Geometry check sheet. Reference: drawing and pictorial views, mm from the part's lowest x, y, z. A direction names the side the tool comes from. Coordinates: 2 decimals unless noted, no trailing zeros. Loops run counter-clockwise (first coordinate to the right, second up) from the corner with the lowest first, then second, coordinate; pieces in that order, holes last. Notation, with made-up numbers: (47.5, 59) -> (55.5, 59) arc R8 cw to (55.5, 70) -> close; hole circle Ø10 at (30, 75). An arc over 180 degrees is marked (long way). Answer as a JSON object with one key per item and string values. Group by question number.
Q1. Cross-section at A-A on y = 7. Give the number of separate pieces and of enclosed holes in the cut face, and give its area (3 significant figures).
Q2. Gauge pin test, flat ends, axial feed: pin 1 Ø2 at (x, z) = (3, 6) entering from -Y; pin 2 Ø6.5 at (x, y) = (5.5, 13.5) entering from -Z; pin 3 Ø2.5 at (y, z) = (17.5, 5.5) entering from +X; pin 4 Ø2 at (y, z) = (10, 2) entering from -X. Record the tip position at first contact, or that the pin passes through.
Q3. Set-up check for the marked faces 1 and 2: record each of +Z, -Z, +X, -X, +Y, -Y from which the full face is reachable in a straight line by a thin tool's end or side.
Q4. Cross-section at C-C on x = 3. Record the boundary of the cut face in (y, z).
Q5. Cross-section at B-B on z = 1. Record the boundary of the cut face in (x, y), and give its area (3 significant figures).
Q6. Cross-section at D-D on x = 9.5. Record the boundary of the cut face in (y, z), and give its area (3 significant figures).
Q7. Scan lines: L1, parallel to Y at x = 16.25, z = 4.75; L2, parallel to Z at x = 13, y = 19.65; L3, parallel to X at y = 7, z = 7. Record each from-to range of solid material in increasing order.
Q8. Release check for a two-part mould opening along Z. For the marked faces 3, 4 and 5 record: released by +Z, released by -Z, zero draft, split by the parting line, or undercut.
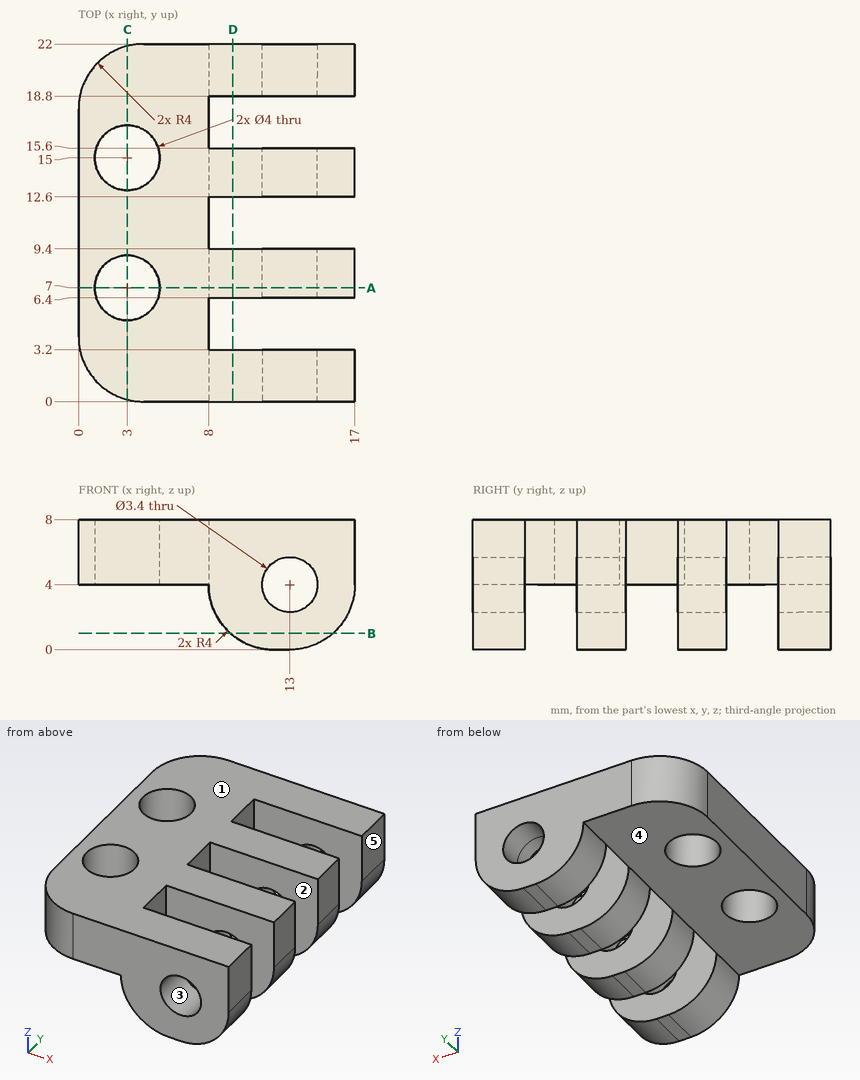
Computed values:
{
 "1": {"separate pieces": "2", "enclosed holes": "1", "area": "72.1 mm²"},
 "2": {"pin 1": "stops at y = 0", "pin 2": "stops at z = 1.67", "pin 3": "stops at x = 8", "pin 4": "stops at x = 8.18"},
 "3": {"face 1": "+Z, +X, -X, +Y, -Y", "face 2": "+Z, -Z, +X"},
 "4": {"outline": "(0.13, 4) -> (5, 4) -> (5, 8) -> (0.13, 8) -> close; (9, 4) -> (13, 4) -> (13, 8) -> (9, 8) -> close; (17, 4) -> (21.87, 4) -> (21.87, 8) -> (17, 8) -> close"},
 "5": {"outline": "(9.35, 0) -> (15.65, 0) -> (15.65, 3.2) -> (9.35, 3.2) -> close; (9.35, 6.4) -> (15.65, 6.4) -> (15.65, 9.4) -> (9.35, 9.4) -> close; (9.35, 12.6) -> (15.65, 12.6) -> (15.65, 15.6) -> (9.35, 15.6) -> close; (9.35, 18.8) -> (15.65, 18.8) -> (15.65, 22) -> (9.35, 22) -> close", "area": "78.0 mm²"},
 "6": {"outline": "(0, 0.88) -> (3.2, 0.88) -> (3.2, 8) -> (0, 8) -> close; (6.4, 0.88) -> (9.4, 0.88) -> (9.4, 8) -> (6.4, 8) -> close; (12.6, 0.88) -> (15.6, 0.88) -> (15.6, 8) -> (12.6, 8) -> close; (18.8, 0.88) -> (22, 0.88) -> (22, 8) -> (18.8, 8) -> close", "area": "88.3 mm²"},
 "7": {"L1": "y = 0 to 3.2, 6.4 to 9.4, 12.6 to 15.6, 18.8 to 22", "L2": "z = 0 to 2.3, 5.7 to 8", "L3": "x = 0 to 1, 5 to 17"},
 "8": {"face 3": "undercut", "face 4": "released by -Z", "face 5": "zero draft"}
}
